```python
from build123d import *

# Parameters (mm, degrees)
BOSS_EXTRUDE1_DEPTH = 82.55
CHAMFER1_SIZE       = 25.4


with BuildPart() as part:
    # Sketch1 → Boss-Extrude1 (new body)
    with BuildSketch(Plane.XY):
        Polygon((0, 25.4), (0, 0), (25.4, 0), (25.4, 3.175), (3.175, 3.175), (3.175, 25.4), align=None)
    extrude(amount=BOSS_EXTRUDE1_DEPTH)

    # Chamfer1
    chamfer1_edges = [part.edges().sort_by_distance(p)[0] for p in [
        (1.5875, 25.4, 0),
        (1.5875, 25.4, 82.55),
    ]]
    chamfer(chamfer1_edges, length=CHAMFER1_SIZE - 0.0001)  # a hair under: the kernel refuses the full size


solid = part.part
```
The listing builds one solid part. Answer for the finished solid, in the listing's coordinates (mm). A direction names the side the tool comes from. Coordinates: 2 decimals unless noted, no trailing zeros. Write each loop counter-clockwise with the first axis right and the second up, starting at its lowest first coordinate (ties: lowest second). Pieces come first, ordered by that corner, then holes. Notation, with made-up numbers: (14.25, 41) - (28.25, 41) arc R9 ccw to (28.25, 52) - close; hole circle Ø11 at (-10.5, -11.5). An arc over 180 degrees is marked (long way). One line per item, written item: value.
1) Find section A-A (z = 31). Give the vertices of the cut face in (x, y) (3 decimals).
Geometry check:
outline: (0, 0) - (25.4, 0) - (25.4, 3.175) - (3.175, 3.175) - (3.175, 25.4) - (0, 25.4) - close
2) Find section C-C (y = 5.25). Give the vertices of the cut face in (x, z) (3 decimals), and give its area (3 significant figures).
Geometry check:
outline: (0, 5.25) - (3.175, 5.25) - (3.175, 77.3) - (0, 77.3) - close
area: 229 mm2
3) Consider line 1 along Y through (x, z) = (11.25, 10.5) (3 decimals); line 2 along Z through (x, y) = (19, 2). Determine where each line is inside the solid, lowest interval first. Write a range as from..to.
Geometry check:
line 1: y = 0..3.175
line 2: z = 2..80.55
4) Each of these flat-tipped pins is pushed along its axis until it touches: pin 1 Ø6.5 at (x, z) = (16, 33) entering from +Y (3 decimals); pin 2 Ø11 at (y, z) = (14.5, 52.5) entering from +X (3 decimals); pin 3 Ø10 at (x, z) = (6.5, 57.5) entering from +Y. Where does it stop, or does it pass through?
Geometry check:
pin 1: stops at y = 3.175
pin 2: stops at x = 3.175
pin 3: stops at y = 25.4
5) A tool of negligible diameter and unlimited length cuts with its end or side. For faces 1 (the flat face through (14, 3.175, 41)), 2 (the flat face through (2, 25.4, 41)), from which of +Z, -Z, +X, -X, +Y, -Y can it reach the whole face along a straight path? Write none if from no direction.
Geometry check:
face 1: +Z, -Z, +X, +Y
face 2: +Z, -Z, +X, -X, +Y
6) Find section D-D (y = 17.25). Give the vertices of the cut face in (x, z) (3 decimals).
Geometry check:
outline: (0, 17.25) - (3.175, 17.25) - (3.175, 65.3) - (0, 65.3) - close
